```python
from build123d import *

# Parameters (mm, degrees)
SKETCH1_R           = 7
SKETCH1_R_2         = 5
BOSS_EXTRUDE1_DEPTH = 12
SKETCH2_R           = 9
SKETCH2_R_2         = 5
BOSS_EXTRUDE2_DEPTH = 2
FILLET1_R           = 0.3


with BuildPart() as part:
    # Sketch1 → Boss-Extrude1 (new body)
    with BuildSketch(Plane(origin=(0, 0, 0), x_dir=(0, 0, -1), z_dir=(1, 0, 0))):
        Circle(SKETCH1_R)
        Circle(SKETCH1_R_2, mode=Mode.SUBTRACT)
    extrude(amount=-BOSS_EXTRUDE1_DEPTH)

    # Sketch2 → Boss-Extrude2 (add)
    with BuildSketch(Plane.ZY.offset(12)):
        Circle(SKETCH2_R)
        with Locations(Location((0, 0, 0), (0, 0, 180))):
            Circle(SKETCH2_R_2, mode=Mode.SUBTRACT)
    extrude(amount=BOSS_EXTRUDE2_DEPTH)

    # Fillet1
    fillet1_edges = [part.edges().sort_by_distance(p)[0] for p in [
        (-12, 0, 7),
        (-14, 0, -9),
        (0, 0, 7),
    ]]
    fillet(fillet1_edges, radius=FILLET1_R)


solid = part.part
```
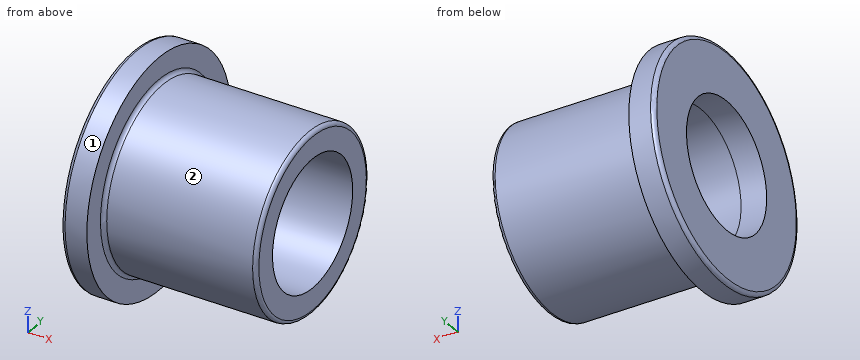
Can you work these out from the model? Positions are in its coordinate system, mm. Face numbers are marked on the shaded views. A direction names the side the tool comes from. Round coordinates to 2 decimals unless told otherwise and drop trailing zeros. Loops run counter-clockwise (first coordinate to the right, second up) from the corner with the lowest first, then second, coordinate; pieces in that order, holes last.
Item 1: Please list where these lines run through material, in increasing order: L1, parallel to Y at x = -3.75, z = 0; L2, parallel to Z at x = -0.75, y = -3.5; L3, parallel to Z at x = -4, y = 3.
Item 2: Which directions (+Z, -Z, +X, -X, +Y, -Y) give clear straight access to the entire face, cutting with the end or side of a thin tool? Please do the marked faces 1 and 2.
Item 3: Suppose I cut it at B-B, the plane x = -8.5. Write out the boundary of the cut face in (y, z).
Item 4: Suppose I cut it at A-A, the plane z = 0. Write out the boundary of the cut face in (x, y).
Item 5: Will these pins go through, and if not, where does the flat tip stop? pin 1 Ø2 at (x, y) = (-2, -2) entering from +Z; pin 2 Ø4 at (x, y) = (-10.5, -5.5) entering from +Z; pin 3 Ø2 at (x, y) = (-8.5, 3.5) entering from +Z.
Reported:
1. L1: y = -7 to -5, 5 to 7
1. L2: z = -6.06 to -3.57, 3.57 to 6.06
1. L3: z = -6.32 to -4, 4 to 6.32
2. face 1: +X, -X
2. face 2: +X
3. outline: circle Ø14 at (0, 0); hole circle Ø10 at (0, 0)
4. outline: (-14, -8.7) arc R0.3 ccw to (-13.7, -9) - (-12, -9) - (-12, -7.3) arc R0.3 cw to (-11.7, -7) - (-0.3, -7) arc R0.3 ccw to (0, -6.7) - (0, -5) - (-14, -5) - close; (-14, 5) - (0, 5) - (0, 6.7) arc R0.3 ccw to (-0.3, 7) - (-11.7, 7) arc R0.3 cw to (-12, 7.3) - (-12, 9) - (-13.7, 9) arc R0.3 ccw to (-14, 8.7) - close
5. pin 1: stops at z = 6.93
5. pin 2: stops at z = 7.97
5. pin 3: stops at z = 6.54
